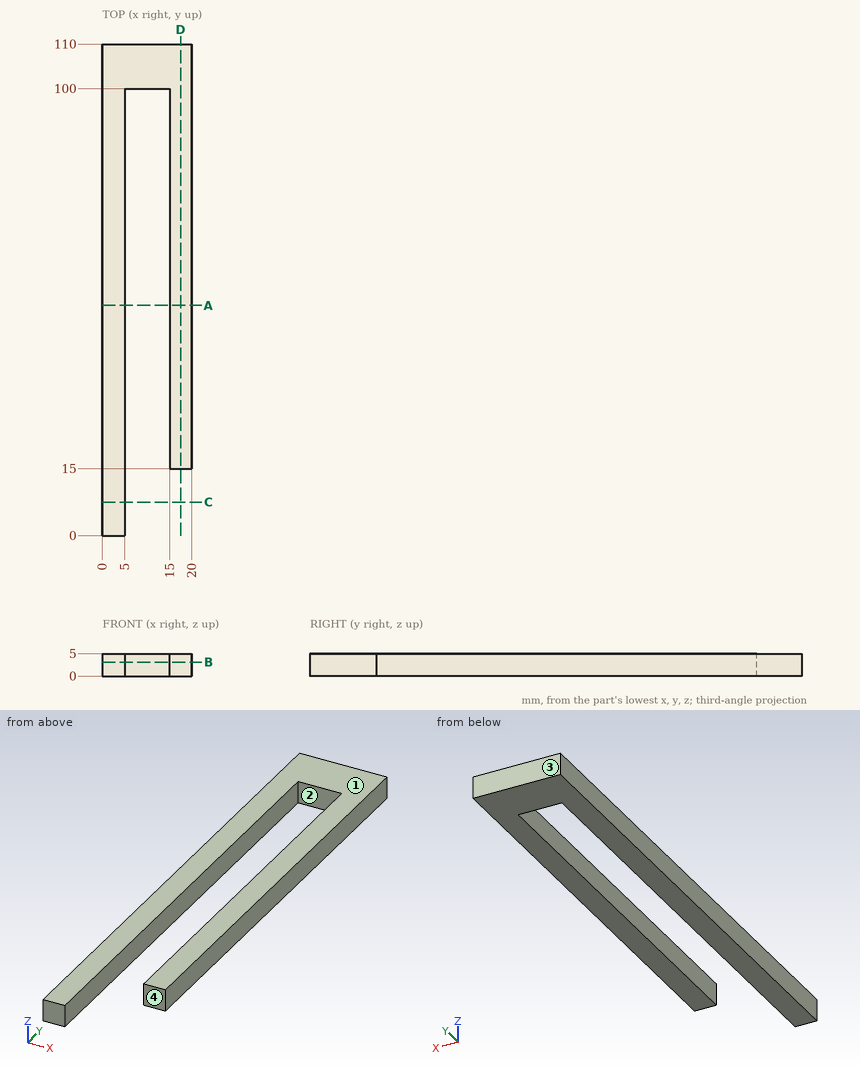
Answer from the drawing. Dimensions are ordinates in mm from the lowest x, y and z of the part. A direction names the side the tool comes from. Coordinates: 2 decimals unless noted, no trailing zeros. Loops run counter-clockwise (first coordinate to the right, second up) from the corner with the lowest first, then second, coordinate; pieces in that order, holes last. Notation, with made-up numbers: (-7.75, 0) - (-2.75, 0) arc R7 cw to (-2.75, 8) - close; hole circle Ø3 at (13.25, 29). An arc over 180 degrees is marked (long way). Use a Markdown table: item, result.
Item 1: Given pin 1 Ø4 at (x, y) = (6.5, 73.5) entering from +Z; pin 2 Ø1 at (x, y) = (13.5, 67) entering from +Z, each flat-ended and moving along its own axis, determine where each tip first touches the part or whether it passes through.
Evaluation:
| item | result |
|---|---|
| pin 1 | stops at z = 5 |
| pin 2 | passes through |
Item 2: Find section A-A, the plane y = 51.5. Determine the outline of the cut face in (x, z).
Evaluation:
| item | result |
|---|---|
| outline | (0, 0) - (5, 0) - (5, 5) - (0, 5) - close; (15, 0) - (20, 0) - (20, 5) - (15, 5) - close |
Item 3: Consider probe 1 along X at (y, z) = (82, 4.1); probe 2 along Y at (x, z) = (14.75, 1.45). Determine where each line is inside the solid, lowest interval first. Write a range as from..to.
Evaluation:
| item | result |
|---|---|
| probe 1 | x = 0..5, 15..20 |
| probe 2 | y = 100..110 |
Item 4: The mould has two halves that part along X. Classify the marked faces 1 and 2: +X half, -X half, draft (parallel to the pull), parting line (faces both ways), or undercut.
Evaluation:
| item | result |
|---|---|
| face 1 | draft |
| face 2 | undercut |
Item 5: For the marked faces 3 and 4, determine the directions among +Z, -Z, +X, -X, +Y, -Y from which every point of the face is accessible in a straight line to the end or side of a thin tool.
Evaluation:
| item | result |
|---|---|
| face 3 | +Z, -Z, +X, -X, +Y |
| face 4 | +Z, -Z, +X, -Y |
Item 6: Find section D-D, the plane x = 17.5. Determine the outline of the cut face in (y, z).
Evaluation:
| item | result |
|---|---|
| outline | (15, 0) - (110, 0) - (110, 5) - (15, 5) - close |
Item 7: Find section B-B, the plane z = 3.1. Determine the outline of the cut face in (x, y), and give its area (4 significant figures).
Evaluation:
| item | result |
|---|---|
| outline | (0, 0) - (5, 0) - (5, 100) - (15, 100) - (15, 15) - (20, 15) - (20, 110) - (0, 110) - close |
| area | 1,125 mm2 |
Item 8: Find section C-C, the plane y = 7.5. Determine the outline of the cut face in (x, z), and give its area (3 significant figures).
Evaluation:
| item | result |
|---|---|
| outline | (0, 0) - (5, 0) - (5, 5) - (0, 5) - close |
| area | 25.0 mm2 |
